```python
from build123d import *

# Parameters (mm, degrees)
F1_DEPTH = 25
F4_DEPTH = 25


# Not quite as in the source:
# - a pattern or mirror of a feature is missing from the dataset's text; its kind, count and spacing are read off the source's solid


with BuildPart() as f1:
    # F0 (on Front) → F1 (new body)
    with BuildSketch(Plane.XZ):
        with BuildLine():
            ThreePointArc((0, 5), (1.4644660941, 1.4644660941), (5, 0))
            Line((5, 0), (25.3563662991, 0))
            Line((25.3563662991, 0), (25.3563662991, 15.7199426368))
            ThreePointArc((25.3563662991, 15.7199426368), (23.891900205, 19.2554765427), (20.3563662991, 20.7199426368))
            Line((20.3563662991, 20.7199426368), (0, 20.7199426368))
            Line((0, 20.7199426368), (0, 5))
        make_face()
    extrude(amount=F1_DEPTH)

    # F2: F1 across face


with BuildPart() as f1_1:
    add(f1.part)
    add(f1.part.mirror(Plane(origin=(15.1781831495, -12.5, 0), x_dir=(1, 0, 0), z_dir=(0, 0, -1))))

    # F3 (on face) → F4 (cut)
    with BuildSketch(Plane(origin=(0, 0, 0), x_dir=(-1, 0, 0), z_dir=(0, 1, 0))):
        with BuildLine():
            Line((-20.3563662991, 20.7199426368), (-17.3368447248, 20.7199426368))
            ThreePointArc((-17.3368447248, 20.7199426368), (-21.2996072768, 23.4502367244), (-23.8041703997, 19.34108153))
            ThreePointArc((-23.8041703997, 19.34108153), (-22.2130172536, 20.3624470507), (-20.3563662991, 20.7199426368))
        make_face()
        with BuildLine():
            ThreePointArc((-23.8041703997, 19.34108153), (-20.1700051206, 16.929235893), (-17.2975812754, 20.2115122229))
            ThreePointArc((-17.2975812754, 20.2115122229), (-17.3074117289, 20.4664843313), (-17.3368447248, 20.7199426368))
            Line((-17.3368447248, 20.7199426368), (-20.3563662991, 20.7199426368))
            ThreePointArc((-20.3563662991, 20.7199426368), (-22.2130172536, 20.3624470507), (-23.8041703997, 19.34108153))
        make_face()
    f4 = extrude(amount=-F4_DEPTH, mode=Mode.SUBTRACT)

    # F4_copies: F4 across plane
    add(f4.mirror(Plane(origin=(0, 0, 0), x_dir=(-1, 0, 0), z_dir=(0, 0, -1))), mode=Mode.SUBTRACT)


solid = f1_1.part
```
Check sheet for the modelled part. Datum: model origin and axes. Units: mm. Round coordinates to 2 decimals unless told otherwise and drop trailing zeros. Write each loop counter-clockwise with the first axis right and the second up, starting at its lowest first coordinate (ties: lowest second). Pieces come first, ordered by that corner, then holes. Notation, with made-up numbers: M 13,78.5 L 39,78.5 A23 cw 39,97.5 Z; hole C 3,16.5 d10. An arc over 180 degrees is marked long. Write item = value, one per line. Start each with the question number.
1. Release check for a two-part mould opening along Z. For faces 1 (the cylindrical face through (1, -12, -2)), 2 (the flat face through (0, -12, -13)), 3 (the cylindrical face through (24.963, -12.325, -17.664)) record: pulls with the +Z half, pulls with the -Z half, needs draft (parallel to the pull), parting line crosses it, or undercut.
2. Section check D-D, the plane x = 18. Record the cut outline in (y, z), then the cut area to 3 significant figures.
3. Scan lines: line 1 (X direction, y = -12.5, z = 19); line 2 (Z direction, x = 18.75, y = -10.75); line 3 (X direction, y = -13.5, z = -4). Record each from-to range of solid material in increasing order. Write a range as [from, to].
4. Section check A-A, the plane y = -17.75. Record the cut outline in (x, z).
5. Section check C-C, the plane x = 21. Record the cut outline in (y, z).
6. Section check B-B, the plane x = 1.5. Record the cut outline in (y, z), then the cut area to 3 significant figures.
7. Gauge pin test, flat ends, axial feed: pin 1 (1 mm diameter, centred on x = 20, y = -18, fed in from +Z); pin 2 (4 mm diameter, centred on y = -3.5, z = 1, fed in from -X). Record the tip position at first contact, or that the pin passes through.
Results found:
q1.face_1 = undercut
q1.face_2 = needs draft
q1.face_3 = pulls with the -Z half
q2.outline = M -25,-18.17 L 0,-18.17 L 0,18.17 L -25,18.17 Z
q2.area = 909 mm^2
q3.line_1 = [0, 17.53], [23.69, 24.13]
q3.line_2 = [-17.47, 17.47]
q3.line_3 = [0.1, 25.36]
q4.outline = M 0,-20.72 L 17.34,-20.72 A3.31 cw 23.8,-19.34 A5 ccw 25.36,-15.72 L 25.36,15.72 A5 ccw 23.8,19.34 A3.31 cw 17.34,20.72 L 0,20.72 L 0,5 A5 ccw 5,0 A5 ccw 0,-5 Z
q5.outline = M -25,-16.92 L 0,-16.92 L 0,16.92 L -25,16.92 Z
q6.outline = M -25,-20.72 L 0,-20.72 L 0,-1.43 L -25,-1.43 Z; M -25,1.43 L 0,1.43 L 0,20.72 L -25,20.72 Z
q6.area = 965 mm^2
q7.pin_1 = 17.09
q7.pin_2 = 0.42
